```python
from build123d import *

# Parameters (mm, degrees)
SKETCH_1_R               = 5.025
EXTRUDE_1_DEPTH          = 3
SKETCH_2_R               = 1.6
SKETCH_2_R_2             = 10.25
SKETCH_2_R_3             = 14
CUT_EXTRUDE_1_DEPTH      = 130.55693729
EXTRUDE_START            = -3
EXTRUDE_2_DEPTH          = 3
SKETCH_3_R               = 1.5
SKETCH_3_W               = 46
SKETCH_3_H               = 5
CUT_EXTRUDE_2_DEPTH      = 135.433749111
CUT_EXTRUDE_3_DEPTH      = 135.433749111
CUT_EXTRUDE_3_DEPTH_BACK = 135.433749111
SKETCH_5_R               = 1
SKETCH_6_R               = 5
CUT_EXTRUDE_5_DEPTH      = 135.433749111
FILLET_1_R               = 1


with BuildPart() as part:
    # ｽｹｯﾁ1 → ﾎﾞｽ - 押し出し1 (new body)
    with BuildSketch(Plane.XY):
        with BuildLine():
            Line((96, -30), (-96, -30))
            ThreePointArc((-96, -30), (-126, 0), (-96, 30))
            Line((-96, 30), (96, 30))
            ThreePointArc((96, 30), (126, 0), (96, -30))
        make_face()
        with Locations((-96, 0)):
            Circle(SKETCH_1_R, mode=Mode.SUBTRACT)
        with Locations((96, 0)):
            Circle(SKETCH_1_R, mode=Mode.SUBTRACT)
    extrude(amount=EXTRUDE_1_DEPTH)

    # ｽｹｯﾁ2 → ｶｯﾄ - 押し出し1 (cut, through all)
    with BuildSketch(Plane.XY.offset(3)):
        with Locations((-59.307299254, 5.75)):
            Circle(SKETCH_2_R)
        with Locations((-59.307299254, -16.25)):
            Circle(SKETCH_2_R)
        with Locations((-19.307299254, -16.25)):
            Circle(SKETCH_2_R)
        with Locations((-19.307299254, 5.75)):
            Circle(SKETCH_2_R)
        with Locations(Location((19.307299254, 5.75, 0), (0, 0, 180))):
            Circle(SKETCH_2_R)
        with Locations(Location((19.307299254, -16.25, 0), (0, 0, 180))):
            Circle(SKETCH_2_R)
        with Locations(Location((59.307299254, 5.75, 0), (0, 0, 180))):
            Circle(SKETCH_2_R)
        with Locations(Location((59.307299254, -16.25, 0), (0, 0, 180))):
            Circle(SKETCH_2_R)
        with Locations((51.307299254, -5.25)):
            Circle(SKETCH_2_R_2)
        with Locations((-51.307299254, -5.25)):
            Circle(SKETCH_2_R_2)
        with Locations((-70.5, 25)):
            Circle(SKETCH_2_R)
        with Locations((0, -2.25)):
            Circle(SKETCH_2_R_3)
        with Locations((-70.5, -25)):
            Circle(SKETCH_2_R)
        with Locations(Location((70.5, -25, 0), (0, 0, 180))):
            Circle(SKETCH_2_R)
        with Locations(Location((70.5, 25, 0), (0, 0, 180))):
            Circle(SKETCH_2_R)
    extrude(amount=-CUT_EXTRUDE_1_DEPTH, mode=Mode.SUBTRACT)

    # ｽｹｯﾁ4 → ﾎﾞｽ - 押し出し2 (add)
    with BuildSketch(Plane.XY.offset(3).offset(EXTRUDE_START)):
        with BuildLine():
            Line((-124.26065672, 10.06654269), (-120.611311687, 20.311657664))
            ThreePointArc((-120.611311687, 20.311657664), (-106.051810297, 39.489926307), (-83.1, 46.77))
            Line((-83.1, 46.77), (83.1, 46.77))
            ThreePointArc((83.1, 46.77), (106.051810297, 39.489926307), (120.611311687, 20.311657664))
            Line((120.611311687, 20.311657664), (124.26065672, 10.06654269))
            ThreePointArc((124.26065672, 10.06654269), (113.291670239, 24.515263416), (96, 30))
            Line((96, 30), (-96, 30))
            ThreePointArc((-96, 30), (-113.291670239, 24.515263416), (-124.26065672, 10.06654269))
        make_face()
        with BuildLine():
            Line((-84.297970262, -31.75), (84.297970262, -31.75))
            ThreePointArc((84.297970262, -31.75), (94.651109882, -30.980141557), (104.776522304, -28.6875))
            ThreePointArc((104.776522304, -28.6875), (100.437059837, -29.670060667), (96, -30))
            Line((96, -30), (-96, -30))
            ThreePointArc((-96, -30), (-100.437059837, -29.670060667), (-104.776522304, -28.6875))
            ThreePointArc((-104.776522304, -28.6875), (-94.651109882, -30.980141557), (-84.297970262, -31.75))
        make_face()
    extrude(amount=EXTRUDE_2_DEPTH)

    # ｽｹｯﾁ3 → ｶｯﾄ - 押し出し2 (cut, through all)
    with BuildSketch(Plane.XY.offset(3)):
        with Locations((-61.057299254, 37.02)):
            Circle(SKETCH_3_R)
        with Locations(Location((-9.057299254, 37.02, 0), (0, 0, 180))):
            Circle(SKETCH_3_R)
        with Locations((-9.057299254, -22)):
            Circle(SKETCH_3_R)
        with Locations(Location((-61.057299254, -22, 0), (0, 0, 180))):
            Circle(SKETCH_3_R)
        with Locations((61.057299254, -22)):
            Circle(SKETCH_3_R)
        with Locations(Location((9.057299254, -22, 0), (0, 0, 180))):
            Circle(SKETCH_3_R)
        with Locations((9.057299254, 37.02)):
            Circle(SKETCH_3_R)
        with Locations(Location((61.057299254, 37.02, 0), (0, 0, 180))):
            Circle(SKETCH_3_R)
        with Locations((-35.057299254, 37.02)):
            Rectangle(SKETCH_3_W, SKETCH_3_H)
        with Locations((-35.057299254, -22)):
            Rectangle(SKETCH_3_W, SKETCH_3_H)
        with Locations((35.057299254, -22)):
            Rectangle(SKETCH_3_W, SKETCH_3_H)
        with Locations((35.057299254, 37.02)):
            Rectangle(SKETCH_3_W, SKETCH_3_H)
    extrude(amount=-CUT_EXTRUDE_2_DEPTH, mode=Mode.SUBTRACT)

    # ｽｹｯﾁ5 → ｶｯﾄ - 押し出し3 (cut, two sides: drawn at the far end of the back side and taken through both)
    with BuildSketch(Plane.XY.offset(3).offset(-CUT_EXTRUDE_3_DEPTH_BACK)):
        with Locations((-58.057299254, 39.52)):
            Circle(SKETCH_5_R)
        with Locations((-58.057299254, 34.52)):
            Circle(SKETCH_5_R)
        with Locations((-12.057299254, 39.52)):
            Circle(SKETCH_5_R)
        with Locations((-12.057299254, 34.52)):
            Circle(SKETCH_5_R)
        with Locations((12.057299254, 34.52)):
            Circle(SKETCH_5_R)
        with Locations((12.057299254, 39.52)):
            Circle(SKETCH_5_R)
        with Locations((58.057299254, 34.52)):
            Circle(SKETCH_5_R)
        with Locations((58.057299254, 39.52)):
            Circle(SKETCH_5_R)
        with Locations((58.057299254, -24.5)):
            Circle(SKETCH_5_R)
        with Locations((58.057299254, -19.5)):
            Circle(SKETCH_5_R)
        with Locations((12.057299254, -24.5)):
            Circle(SKETCH_5_R)
        with Locations((12.057299254, -19.5)):
            Circle(SKETCH_5_R)
        with Locations((-12.057299254, -19.5)):
            Circle(SKETCH_5_R)
        with Locations((-12.057299254, -24.5)):
            Circle(SKETCH_5_R)
        with Locations((-58.057299254, -19.5)):
            Circle(SKETCH_5_R)
        with Locations((-58.057299254, -24.5)):
            Circle(SKETCH_5_R)
    extrude(amount=CUT_EXTRUDE_3_DEPTH + CUT_EXTRUDE_3_DEPTH_BACK, mode=Mode.SUBTRACT)

    # ｽｹｯﾁ6 → ｶｯﾄ - 押し出し5 (cut, through all)
    with BuildSketch(Plane.XY.offset(3)):
        with Locations((0, 14)):
            Circle(SKETCH_6_R)
    extrude(amount=-CUT_EXTRUDE_5_DEPTH, mode=Mode.SUBTRACT)

    # ﾌｨﾚｯﾄ1
    fillet_1_edges = [part.edges().sort_by_distance(p)[0] for p in [
        (4.098852037, 11.136538462, 1.5),
        (-4.098852037, 11.136538462, 1.5),
    ]]
    fillet(fillet_1_edges, radius=FILLET_1_R)


solid = part.part
```
The model under review builds one solid part; all positions refer to its coordinate system, in mm. Give positions to 0.01 mm unless a question says otherwise; leave off trailing zeros. Write each loop counter-clockwise with the first axis right and the second up, starting at its lowest first coordinate (ties: lowest second). Pieces come first, ordered by that corner, then holes. Notation, with made-up numbers: M 41.5,-28 L 91.5,-28 A18 ccw 91.5,6 Z; hole C 26.25,-20.5 d6. An arc over 180 degrees is marked long. Write each question's results on one line, items separated by ' | '. Start each with the question number.
1. We need section B-B (x = 32). Write out the cut boundary in (y, z).
2. We need section D-D (y = -12.5). Write out the cut boundary in (x, z).
3. Mouldability with a two-part tool opening along X and no side actions: class faces 1 (the cylindrical face through (122.954, -13.172, 1.479)), 2 (the flat face through (2, 26, 0)), 3 (the cylindrical face through (-101.02, 0.22, 1.48)), 4 (the cylindrical face through (-0.54, -16.24, 1.52)) as released by +X, released by -X, zero draft, split by the parting line, or undercut.
4. Insertion check: pin 1 Ø1.8 at (x, y) = (58.06, 39.52) entering from -Z. The pin has a flat end and moves straight along its axis. Give the tip position at first contact, or say it passes through.
5. We need section C-C (y = -2.25). Write out the cut boundary in (x, z), and give its area (3 significant figures).
6. For probe 1 along Y at (x, z) = (-28, 2.3); probe 2 along Y at (x, z) = (-12.5, 2.6); probe 3 along X at (y, z) = (5.5, 2.45), list the stretches that pass through material, from the lowest coordinate up. Write a range as [from, to].
7. We need section A-A (x = 0). Write out the cut boundary in (y, z), and give its area (3 significant figures).
Results found:
1) outline: M -31.75,0 L -24.5,0 L -24.5,3 L -31.75,3 Z; M -19.5,0 L 34.52,0 L 34.52,3 L -19.5,3 Z; M 39.52,0 L 46.77,0 L 46.77,3 L 39.52,3 Z
2) outline: M -123.27,0 L -58.55,0 L -58.55,3 L -123.27,3 Z; M -44.06,0 L -9.54,0 L -9.54,3 L -44.06,3 Z; M 9.54,0 L 44.06,0 L 44.06,3 L 9.54,3 Z; M 58.55,0 L 123.27,0 L 123.27,3 L 58.55,3 Z
3) face 1: released by +X | face 2: zero draft | face 3: undercut | face 4: undercut
4) pin 1: passes through
5) outline: M -125.92,0 L -100.49,0 L -100.49,3 L -125.92,3 Z; M -91.51,0 L -61.11,0 L -61.11,3 L -91.51,3 Z; M -41.51,0 L -14,0 L -14,3 L -41.51,3 Z; M 14,0 L 41.51,0 L 41.51,3 L 14,3 Z; M 61.11,0 L 91.51,0 L 91.51,3 L 61.11,3 Z; M 100.49,0 L 125.92,0 L 125.92,3 L 100.49,3 Z | area: 500 mm^2
6) probe 1: y = [-31.75, -24.5], [-19.5, 34.52], [39.52, 46.77] | probe 2: y = [-31.75, -25.4], [-18.6, -8.55], [4.05, 33.62], [40.42, 46.77] | probe 3: x = [-125.49, -60.89], [-57.73, -20.89], [-17.73, -11.66], [11.66, 17.73], [20.89, 57.73], [60.89, 125.49]
7) outline: M -31.75,0 L -16.25,0 L -16.25,3 L -31.75,3 Z; M 19,0 L 46.77,0 L 46.77,3 L 19,3 Z | area: 130 mm^2
